CAD build for the part. Positions are in the model's coordinates, mm. Give positions to 0.01 mm unless a question says otherwise; leave off trailing zeros. Loops run counter-clockwise (first coordinate to the right, second up) from the corner with the lowest first, then second, coordinate; pieces in that order, holes last.
Autodesk Inventor part; units mm, degrees
ref_plane "YZ Plane" through (0, 0, 0) normal (1, 0, 0) x (0, 1, 0)
ref_plane "XZ Plane" through (0, 0, 0) normal (0, 1, 0) x (-1, 0, 0)
ref_plane "XY Plane" through (0, 0, 0) normal (0, 0, 1) x (1, 0, 0)
sketch "Sketch1" plane through (0, 0, 0) normal (0, 0, 1) x (1, 0, 0)
  line L0 (-245, -403) -> (245, -403)
  line L1 (245, -403) -> (245, 403)
  line L2 (245, 403) -> (-245, 403)
  line L3 (-245, 403) -> (-245, -403)
  line L4 (-245, -403) -> (245, 403) construction
  line L5 (245, -403) -> (-245, 403) construction
  point P0 (0, 0)
  dimension "d0" = 490
  dimension "d1" = 806
extrude "Plate1" add sketch "Sketch1" along normal blind 3
sketch "Sketch2" plane through (0, 0, 0) normal (0, 0, -1) x (-1, 0, 0)
  line L0 (-245, 403) -> (245, 403)
  line L1 (-245, -403) -> (-245, 403)
  line L2 (-225, 383) -> (-25, 383) construction
  line L3 (-25, 383) -> (-25, 363) construction
  line L4 (-25, 363) -> (-225, 363) construction
  line L5 (-225, 363) -> (-225, 383) construction
  point P0 (0, 0)
  dimension "d8" = 200
  dimension "d9" = 20
  dimension "d10" = 20
  dimension "d11" = 20
mark "Mark3"
sketch "Sketch6" plane through (0, 0, 3) normal (0, 0, 1) x (1, 0, 0)
  circle A0 centre (0, 173.1375) radius 44.5
  point P0 (0, 0)
  dimension "d42" = 89
extrude "Cut1" cut sketch "Sketch6" against normal blind 3
equation "\"d43\" = Thickness"
equation "\"d2\" = Thickness"
equation "\"BendReliefWidth\" = Thickness"
equation "\"BendReliefDepth\" = 0.5 * Thickness"
equation "\"CornerReliefSize\" = 4 * Thickness"
equation "\"MinimumRemnant\" = 2 * Thickness"
equation "\"TransitionRadius\" = BendRadius"
equation "\"JacobiRadiusSize\" = BendRadius"
equation "\"GapSize\" = Thickness"
properties part number "TRM 011 bottom main" material "AISI 304"
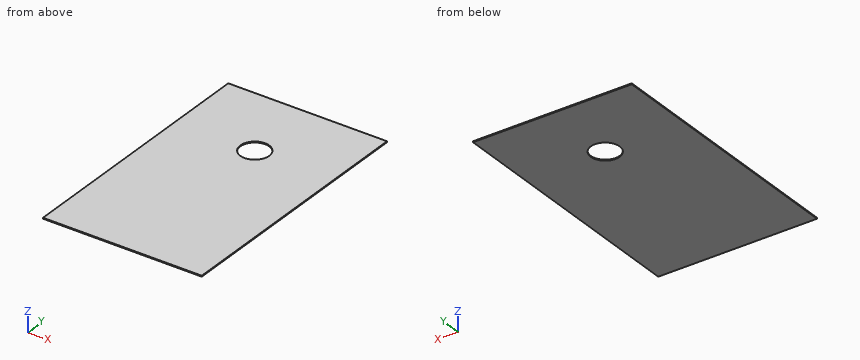
1. Saw through at C-C, the plane z = 0.55. List the corners of the cut face in (x, y).
Responses:
outline: (-245, -403) - (245, -403) - (245, 403) - (-245, 403) - close; hole circle Ø89 at (0, 173.14)
2. Probe line 1 along Y through (x, z) = (0, 0.85); line 2 along Y through (x, z) = (-2, 2.4). List the from-to ranges inside material, lowest first.
Responses:
line 1: y = -403 to 128.64, 217.64 to 403
line 2: y = -403 to 128.68, 217.59 to 403
3. Saw through at A-A, the plane x = 0. List the corners of the cut face in (y, z).
Responses:
outline: (-403, 0) - (128.64, 0) - (128.64, 3) - (-403, 3) - close; (217.64, 0) - (403, 0) - (403, 3) - (217.64, 3) - close
4. Saw through at B-B, the plane y = 194. List the corners of the cut face in (x, z), and give its area (3 significant figures).
Responses:
outline: (-245, 0) - (-39.31, 0) - (-39.31, 3) - (-245, 3) - close; (39.31, 0) - (245, 0) - (245, 3) - (39.31, 3) - close
area: 1,230 mm2
